Autodesk Inventor part; units mm, degrees
ref_plane "YZ Plane" through (0, 0, 0) normal (1, 0, 0) x (0, 1, 0)
ref_plane "XZ Plane" through (0, 0, 0) normal (0, 1, 0) x (-1, 0, 0)
ref_plane "XY Plane" through (0, 0, 0) normal (0, 0, 1) x (1, 0, 0)
ref_plane "작업 평면1" through (0, 0, 0) normal (0, 0, 1) x (1, 0, 0)
sketch "스케치1" plane through (0, 0, 0) normal (0, 0, 1) x (1, 0, 0)
  arc A0 (5.05, 17.3607) -> (6.05, 18.3607) centre (6.05, 17.3607) ccw
  line L0 (5.05, 17.3607) -> (-5.05, 17.3607)
  arc A1 (-6.05, 18.3607) -> (-5.05, 17.3607) centre (-6.05, 17.3607) ccw
  line L1 (-6.05, 18.3607) -> (-6.05, 23.4607)
  line L2 (-6.05, 23.4607) -> (-20.8, 23.4607)
  line L3 (-20.8, 23.4607) -> (-20.8, -2.5393)
  line L4 (-20.8, -2.5393) -> (-10.8995, -13.2319)
  arc A2 (-10.8995, -13.2319) -> (-5.5649, -22.7117) centre (0, -13.3393) ccw
  arc A3 (-5.5649, -22.7117) -> (-4.0544, -21.8465) centre (-5.0543, -21.8519) ccw
  line L5 (-4.0544, -21.8465) -> (-4.0998, -13.3833)
  arc A4 (4.1, -13.3393) -> (-4.0998, -13.3833) centre (0, -13.3393) ccw
  line L6 (4.1, -13.3393) -> (4.1, -21.8246)
  arc A5 (4.1, -21.8246) -> (5.6152, -22.6817) centre (5.1, -21.8246) ccw
  arc A6 (5.6152, -22.6817) -> (10.8995, -13.2319) centre (0, -13.3393) ccw
  line L7 (10.8995, -13.2319) -> (20.8, -2.5393)
  line L8 (20.8, -2.5393) -> (20.8, 23.4607)
  line L9 (20.8, 23.4607) -> (6.05, 23.4607)
  line L10 (6.05, 23.4607) -> (6.05, 18.3607)
  circle A7 centre (5.6569, -18.9962) radius 1.2
  circle A8 centre (5.6569, -7.6825) radius 1.2
  circle A9 centre (-5.6569, -7.6825) radius 1.2
  circle A10 centre (0, -5.3393) radius 1.2
  circle A11 centre (8, -13.3393) radius 1.2
  circle A12 centre (-15.8, 20.4107) radius 1.35
  circle A13 centre (15.8, 20.4107) radius 1.35
  circle A14 centre (-8, -13.3393) radius 1.2
  circle A15 centre (-5.6569, -18.9962) radius 1.2
  line L11 (-20.8, 23.4607) -> (20.8, 23.4607)
  line L12 (20.8, 23.4607) -> (20.8, -2.5393)
  line L13 (20.8, -2.5393) -> (-20.8, -2.5393)
  line L14 (-20.8, -2.5393) -> (-20.8, 23.4607)
  circle A16 centre (0, -13.3393) radius 4.1
  circle A17 centre (0, -13.3393) radius 10.9
  circle A18 centre (0, -5.3393) radius 1.2
  circle A19 centre (-5.6569, -7.6825) radius 1.2
  circle A20 centre (-8, -13.3393) radius 1.2
  circle A21 centre (-5.6569, -18.9962) radius 1.2
  circle A22 centre (0, -21.3393) radius 1.2
  circle A23 centre (5.6569, -18.9962) radius 1.2
  circle A24 centre (8, -13.3393) radius 1.2
  circle A25 centre (5.6569, -7.6825) radius 1.2
  line L15 (-20.8, -2.5393) -> (-10.8995, -13.2319)
  line L16 (10.8995, -13.2319) -> (20.8, -2.5393)
  point P0 (0, 0)
  point P1 (-1.4731, -2.5393)
  point P2 (1.4731, -2.5393)
  dimension "d2" = 360
extrude "돌출1" add sketch "스케치1" against normal blind 6 contours L0 A1 L1 L11 L10 A0 | A0 L10 L9 L8 L13 A17 L3 L2 L1 A1 L0 | L7 A17 L13 | A6 A5 L6 A4 L5 A3 A2 A17 L13 | L13 A17 L4 | A12 | A13
sketch "스케치2" plane through (0, 0, -6) normal (0, 0, -1) x (-1, 0, 0)
  circle A0 centre (-5.6569, -18.9962) radius 1.2
  circle A1 centre (-5.6569, -7.6825) radius 1.2
  circle A2 centre (5.6569, -7.6825) radius 1.2
  circle A3 centre (0, -5.3393) radius 1.2
  circle A4 centre (-8, -13.3393) radius 1.2
  circle A5 centre (15.8, 20.4107) radius 1.35
  circle A6 centre (-15.8, 20.4107) radius 1.35
  circle A7 centre (8, -13.3393) radius 1.2
  circle A8 centre (5.6569, -18.9962) radius 1.2
  arc A9 (-6.05, 18.3607) -> (-5.05, 17.3607) centre (-6.05, 17.3607) ccw
  line L0 (-6.05, 18.3607) -> (-6.05, 23.4607)
  line L1 (-20.8, 23.4607) -> (-6.05, 23.4607)
  line L2 (-20.8, -2.5393) -> (-20.8, 23.4607)
  line L3 (-10.8995, -13.2319) -> (-20.8, -2.5393)
  arc A10 (-10.8995, -13.2319) -> (-5.6152, -22.6817) centre (0, -13.3393) ccw
  arc A11 (-5.6152, -22.6817) -> (-4.1, -21.8246) centre (-5.1, -21.8246) ccw
  line L4 (-4.1, -13.3393) -> (-4.1, -21.8246)
  arc A12 (4.0998, -13.3833) -> (-4.1, -13.3393) centre (0, -13.3393) ccw
  line L5 (4.0544, -21.8465) -> (4.0998, -13.3833)
  arc A13 (4.0544, -21.8465) -> (5.5649, -22.7117) centre (5.0543, -21.8519) ccw
  arc A14 (5.5649, -22.7117) -> (10.8995, -13.2319) centre (0, -13.3393) ccw
  line L6 (20.8, -2.5393) -> (10.8995, -13.2319)
  line L7 (20.8, 23.4607) -> (20.8, -2.5393)
  line L8 (6.05, 23.4607) -> (20.8, 23.4607)
  line L9 (6.05, 23.4607) -> (6.05, 18.3607)
  arc A15 (5.05, 17.3607) -> (6.05, 18.3607) centre (6.05, 17.3607) ccw
  line L10 (5.05, 17.3607) -> (-5.05, 17.3607)
  line L11 (-20.8, 23.4607) -> (20.8, 23.4607)
  line L12 (20.8, 23.4607) -> (20.8, 17.4607)
  line L13 (20.8, 17.4607) -> (-20.8, 17.4607)
  line L14 (-20.8, 17.4607) -> (-20.8, 23.4607)
  point P0 (0, 0)
  dimension "d6" = 6
extrude "돌출2" add sketch "스케치2" along normal blind 20.5 contours A5 | A6 | L0 L11 L9 A15 L13 A9 | A9 L13 L2 L1 L0 | A15 L9 L8 L7 L13
sketch "스케치3" plane through (-20.8, 23.4607, 0) normal (0, 1, 0) x (1, 0, 0)
  line L0 (39.2, 41.4) -> (34, 41.4)
  line L1 (34, 41.4) -> (34, 43.6)
  line L2 (34, 43.6) -> (39.2, 43.6)
  line L3 (39.2, 43.6) -> (39.2, 41.4)
  line L4 (2.4, 11.6) -> (7.6, 11.6)
  line L5 (7.6, 11.6) -> (7.6, 9.4)
  line L6 (7.6, 9.4) -> (2.4, 9.4)
  line L7 (2.4, 9.4) -> (2.4, 11.6)
  line L8 (39.2, 11.6) -> (39.2, 9.4)
  line L9 (39.2, 9.4) -> (34, 9.4)
  line L10 (34, 9.4) -> (34, 11.6)
  line L11 (34, 11.6) -> (39.2, 11.6)
  line L12 (7.6, 41.4) -> (2.4, 41.4)
  line L13 (2.4, 41.4) -> (2.4, 43.6)
  line L14 (2.4, 43.6) -> (7.6, 43.6)
  line L15 (7.6, 43.6) -> (7.6, 41.4)
  line L16 (14.8, 47) -> (-0.2, 47)
  line L17 (-0.2, 47) -> (-0.2, 6)
  line L18 (-0.2, 6) -> (14.8, 6)
  line L19 (14.8, 0) -> (14.8, 6)
  line L20 (26.8, 0) -> (14.8, 0)
  line L21 (26.8, 0) -> (26.8, 6)
  line L22 (26.8, 6) -> (41.8, 6)
  line L23 (41.8, 6) -> (41.8, 47)
  line L24 (41.8, 47) -> (26.8, 47)
  line L25 (26.8, 53) -> (26.8, 47)
  line L26 (14.8, 53) -> (26.8, 53)
  line L27 (14.8, 53) -> (14.8, 47)
  circle A0 centre (20.8, 26.5) radius 6
  circle A1 centre (20.8, 37.5) radius 1.6
  circle A2 centre (13.0218, 34.2782) radius 1.6
  circle A3 centre (9.8, 26.5) radius 1.6
  circle A4 centre (13.0218, 18.7218) radius 1.6
  circle A5 centre (20.8, 15.5) radius 1.6
  circle A6 centre (28.5782, 18.7218) radius 1.6
  circle A7 centre (31.8, 26.5) radius 1.6
  circle A8 centre (28.5782, 34.2782) radius 1.6
  circle A9 centre (20.8, 26.5) radius 6
  circle A10 centre (13.0218, 18.7218) radius 1.35
  circle A11 centre (20.8, 15.5) radius 1.35
  circle A12 centre (28.5782, 18.7218) radius 1.35
  circle A13 centre (31.8, 26.5) radius 1.35
  circle A14 centre (28.5782, 34.2782) radius 1.35
  circle A15 centre (20.8, 37.5) radius 1.35
  circle A16 centre (13.0218, 34.2782) radius 1.35
  circle A17 centre (9.8, 26.5) radius 1.35
  point P0 (20.8, 0)
  dimension "d9" = 2.7
  dimension "d12" = 360
extrude "돌출3" cut sketch "스케치3" against normal blind 20.5 contours A0 | A10 | A11 | A12 | A13 | A17
mirror "미러1" about plane through (0, 20.4607, -26.5) normal (0, 0, -1)
fillet "모깎기1" radius 2 4 edges at (0, 17.4607, -6) (0, 17.4607, -47) (0, 23.4607, -53) (0, 23.4607, 0)
sketch "스케치4" plane through (0, 0, 0) normal (0, 0, 1) x (1, 0, 0)
  line L0 (1.4731, -2.5393) -> (-1.4731, -2.5393)
  arc A0 (1.4731, -2.5393) -> (-1.4731, -2.5393) centre (0, -13.3393) ccw
  line L1 (-1.6142, -2.1682) -> (1.6887, -2.1682)
  line L2 (1.6887, -2.1682) -> (1.6887, -3.0074)
  line L3 (1.6887, -3.0074) -> (-1.6142, -3.0074)
  line L4 (-1.6142, -3.0074) -> (-1.6142, -2.1682)
  point P0 (0, 0)
extrude "돌출4" add sketch "스케치4" against normal blind 6 contours L0 A0 | L1 L2 L3 L4
sketch "스케치5" plane through (4.1, -21.8246, -53) normal (0, 0, -1) x (-1, 0, 0)
  line L0 (2.2483, 20.1118) -> (6.3529, 20.1118)
  line L1 (6.3529, 20.1118) -> (6.3529, 18.3836)
  line L2 (6.3529, 18.3836) -> (2.2483, 18.3836)
  line L3 (2.2483, 18.3836) -> (2.2483, 20.1118)
  point P0 (4.1, 21.8246)
extrude "돌출5" add sketch "스케치5" against normal blind 6
properties part number "shoulder_ver2_new" material "PMMA 플라스틱"
Design review of the part built by this model. Coordinates are the model's own, in mm. A direction names the side the tool comes from. Give positions to 0.01 mm unless a question says otherwise; leave off trailing zeros. Order: outer loops, then holes, each group sorted by start corner. A loop starts at its lowest first (then second) coordinate and runs counter-clockwise, first axis right, second up. Notation, with made-up numbers: (68, 69) - (88, 69) arc R36 ccw to (88, 108) - close; hole circle Ø11 at (62, -10). An arc over 180 degrees is marked (long way). Use a Markdown table: item, result. Add a question column.
(1) Add section C-C on y = 13.5. Give the boundary of the cut face in (x, z), then the cut area to 3 significant figures.
(2) Clearance check with flat-ended pins moving along their axes: P1, Ø1.9, axis at x = 8, y = -13.34, coming from the +Z side; P2, Ø3, axis at x = -12, y = 3, coming from the +Z side; P3, Ø4.5, axis at x = 0, z = -37.5, coming from the -Y side; P4, Ø4, axis at x = -10, z = -43.5, coming from the -Y side. State where each tip first meets the part, or that it passes through.
(3) Add section D-D on z = -26.5. Give the boundary of the cut face in (x, y).
(4) Machinability: for faces 4 (the face through (-6.61, -18.27, -50.04)), 5 (the face through (4.1, -18, -50)), which of the approach directions +Z, -Z, +X, -X, +Y, -Y give a long, thin tool a straight path to every point of the face, cutting with its end or side? Answer none if there is none.
(5) Add section B-B on x = 0. Give the number of separate pieces and of enclosed holes in the cut face, then the cut area to 3 significant figures.
(6) Mouldability with a two-part tool opening along X and no side actions: class faces 1 (the face through (-9.538, -18.615, -2.958)), 2 (the face through (7, -14, -50)), 3 (the face through (0, 1, -6)) as +X half, -X half, draft (parallel to the pull), parting line (faces both ways), or undercut.
(7) Add section A-A on z = -37.5. Give the boundary of the cut face in (x, y), then the cut area to 3 significant figures.
(8) Wall thickness on probe 1 along Z at (x, y) = (11, 0); probe 2 along Y at (x, z) = (0, -50.6); probe 3 along Z at (x, y) = (-7.5, 18): over which ranges is each line inside the solid? List them lowest first. Write a range as [from, to].
Report:
| question | item | result |
|---|---|---|
| 1 | outline | (-20.8, -53) - (20.8, -53) - (20.8, -47) - (-20.8, -47) - close; (-20.8, -6) - (20.8, -6) - (20.8, 0) - (-20.8, 0) - close |
| 1 | area | 499 mm² |
| 2 | P1 | passes through |
| 2 | P2 | stops at z = 0 |
| 2 | P3 | stops at y = 17.46 |
| 2 | P4 | stops at y = 17.4 |
| 3 | outline | (-20.8, 17.46) - (-12.35, 17.46) - (-12.35, 23.46) - (-20.8, 23.46) - close; (-9.65, 17.46) - (-6, 17.46) - (-6, 23.46) - (-9.65, 23.46) - close; (6, 17.46) - (9.65, 17.46) - (9.65, 23.46) - (6, 23.46) - close; (12.35, 17.46) - (20.8, 17.46) - (20.8, 23.46) - (12.35, 23.46) - close |
| 4 | face 4 | +Z, -Z |
| 4 | face 5 | +Z, -Z, -Y |
| 5 | separate pieces | 6 |
| 5 | enclosed holes | 0 |
| 5 | area | 505 mm² |
| 6 | face 1 | -X half |
| 6 | face 2 | undercut |
| 6 | face 3 | draft |
| 7 | outline | (-20.8, 17.46) - (-1.35, 17.46) - (-1.35, 23.46) - (-20.8, 23.46) - close; (1.35, 17.46) - (20.8, 17.46) - (20.8, 23.46) - (1.35, 23.46) - close |
| 7 | area | 233 mm² |
| 8 | probe 1 | z = [-53, -47], [-6, 0] |
| 8 | probe 2 | y = [-9.24, -6.54], [-4.14, 23.46] |
| 8 | probe 3 | z = [-53, -35.6], [-32.96, -20.04], [-17.4, 0] |
